The model under review builds one solid part; all positions refer to its coordinate system, in mm. Coordinates: 2 decimals unless noted, no trailing zeros. Order: outer loops, then holes, each group sorted by start corner. A loop starts at its lowest first (then second) coordinate and runs counter-clockwise, first axis right, second up. Notation, with made-up numbers: (-7.75, -21.75) - (25.25, -21.75) arc R12 ccw to (25.25, 1.25) - close; hole circle Ø4 at (56.25, 8). An arc over 180 degrees is marked (long way). Answer in a Markdown table with one row per item.
```python
from build123d import *

# Parameters (mm, degrees)
SKETCH1_R           = 3.75
BOSS_EXTRUDE1_DEPTH = 5
CUT_EXTRUDE1_DEPTH  = 2
CUT_EXTRUDE2_DEPTH  = 1.5


with BuildPart() as part:
    # Sketch1 → Boss-Extrude1 (new body)
    with BuildSketch(Plane.XY):
        with BuildLine():
            ThreePointArc((0, 22), (-11, 11), (0, 0))
            Line((0, 0), (127, 0))
            ThreePointArc((127, 0), (138, 11), (127, 22))
            Line((127, 22), (0, 22))
        make_face()
        with Locations((0, 11)):
            Circle(SKETCH1_R, mode=Mode.SUBTRACT)
    extrude(amount=BOSS_EXTRUDE1_DEPTH)

    # Sketch2 → Cut-Extrude1 (cut)
    with BuildSketch(Plane.XY.offset(5)):
        with BuildLine():
            ThreePointArc((129.016666667, 21.813558876), (127, 11), (129.016666667, 0.186441124))
            ThreePointArc((129.016666667, 0.186441124), (129.995854312, 0.415820441), (130.95, 0.733671542))
            ThreePointArc((130.95, 0.733671542), (129, 11), (130.95, 21.266328458))
            ThreePointArc((130.95, 21.266328458), (129.995854312, 21.584179559), (129.016666667, 21.813558876))
        make_face()
    extrude(amount=-CUT_EXTRUDE1_DEPTH, mode=Mode.SUBTRACT)

    # Sketch3 → Cut-Extrude2 (cut)
    with BuildSketch(Plane(origin=(0, 0, 0), x_dir=(-1, 0, 0), z_dir=(0, 0, -1))):
        with BuildLine():
            Line((0, 14.75), (-18.25, 14.75))
            ThreePointArc((-18.25, 14.75), (-22, 11), (-18.25, 7.25))
            Line((-18.25, 7.25), (0, 7.25))
            ThreePointArc((0, 7.25), (-3.75, 11), (0, 14.75))
        make_face()
    extrude(amount=-CUT_EXTRUDE2_DEPTH, mode=Mode.SUBTRACT)


solid = part.part
```
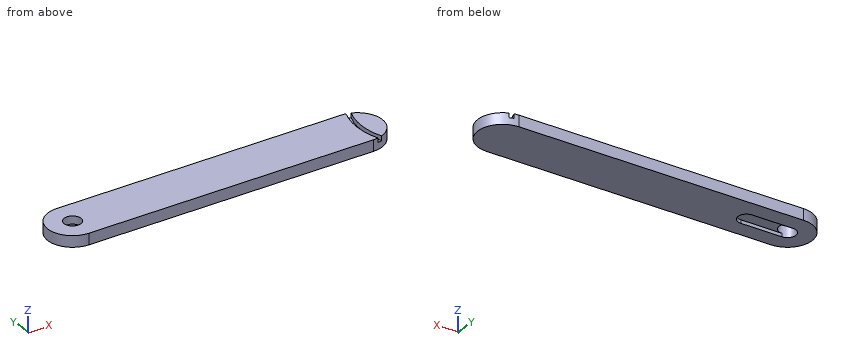
Item 1: We need section C-C, the plane y = 5.5. Write out the cut boundary in (x, z).
Check values:
| item | result |
|---|---|
| outline | (-9.53, 0) - (136.53, 0) - (136.53, 5) - (129.55, 5) - (129.55, 3) - (127.51, 3) - (127.51, 5) - (-9.53, 5) - close |
Item 2: Clearance check with flat-ended pins moving along their axes: pin 1 Ø1.5 at (y, z) = (14, 4) entering from +X; pin 2 Ø2 at (x, y) = (13, 11.5) entering from -Z; pin 3 Ø6 at (x, y) = (0, 11) entering from -Z. State where each tip first meets the part, or that it passes through.
Check values:
| item | result |
|---|---|
| pin 1 | x = 137.77 |
| pin 2 | z = 1.5 |
| pin 3 | through |
Item 3: We need section B-B, the plane y = 11. Write out the cut boundary in (x, z), then the cut area to 3 significant figures.
Check values:
| item | result |
|---|---|
| outline | (-11, 0) - (-3.75, 0) - (-3.75, 5) - (-11, 5) - close; (3.75, 1.5) - (22, 1.5) - (22, 0) - (138, 0) - (138, 5) - (129, 5) - (129, 3) - (127, 3) - (127, 5) - (3.75, 5) - close |
| area | 676 mm^2 |
Item 4: We need section A-A, the plane z = 4. Write out the cut boundary in (x, y).
Check values:
| item | result |
|---|---|
| outline | (0, 0) - (127, 0) arc R11 ccw to (129.02, 0.19) arc R30 cw to (129.02, 21.81) arc R11 ccw to (127, 22) - (0, 22) arc R11 ccw to start; (130.95, 0.73) arc R11 ccw to (130.95, 21.27) arc R28 ccw to start; hole circle Ø7.5 at (0, 11) |
Item 5: To check wall thickness, follow line 1 (X direction, y = 11, z = 2.15); line 2 (X direction, y = 11, z = 3.8); line 3 (X direction, y = 9, z = 3.3). State the ranges of each line that lie inside material, in increasing order. Write a range as from..to.
Check values:
| item | result |
|---|---|
| line 1 | -11..-3.75, 3.75..138 |
| line 2 | -11..-3.75, 3.75..127, 129..138 |
| line 3 | -10.82..-3.17, 3.17..127.07, 129.07..137.82 |
